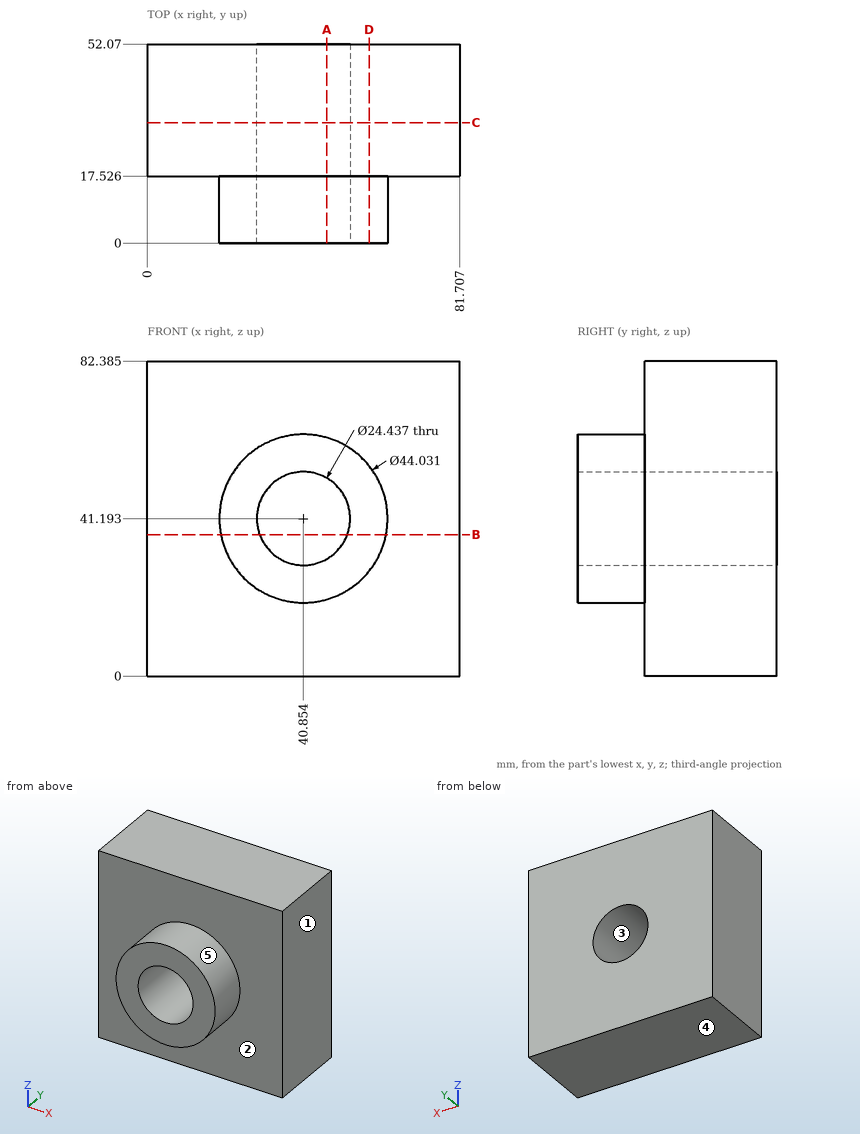
Check sheet for the drawn part. Datum: minimum x, y, z corner. Units: mm. A direction names the side the tool comes from. Round coordinates to 2 decimals unless told otherwise and drop trailing zeros. Order: outer loops, then holes, each group sorted by start corner. A loop starts at its lowest first (then second) coordinate and runs counter-clockwise, first axis right, second up. Notation, with made-up numbers: M 50,50.25 L 99,50.25 A33 ccw 99,80.25 Z; hole C -5,-6.75 d4. An arc over 180 degrees is marked long. Write each question's results on one line, items separated by ' | '. Start each with the question number.
1. Cross-section at B-B on z = 37. Record the boundary of the cut face in (x, y).
2. Cross-section at C-C on y = 31.5. Record the boundary of the cut face in (x, z) (1 decimal).
3. Go/stop test with flat-tipped pins: P1, Ø12, axis at x = 29.5, y = 5.5, coming from the +Z side; P2, Ø10, axis at x = 49.5, z = 40, coming from the -Y side; P3, Ø2, axis at x = 32, y = 11, coming from the -Z side (1 decimal); P4, Ø1, axis at x = 50, z = 63.5, coming from the -Y side. Record where each tip stops, or that it passes through.
4. Cross-section at A-A on x = 47. Record the boundary of the cut face in (y, z) (1 decimal).
5. Material ranges on L1, parallel to Y at x = 57, z = 21; L2, parallel to Z at x = 50, y = 13 (1 decimal); L3, parallel to X at y = 13, z = 46.5, recorded low to high. Write a range as from..to.
6. Set-up check for the marked faces 1 and 2: record each of +Z, -Z, +X, -X, +Y, -Y from which the full face is reachable in a straight line by a thin tool's end or side.
7. Draft check along Z on the marked faces 3, 4 and 5. Enter one of: pulls with the +Z half, pulls with the -Z half, needs draft (parallel to the pull), parting line crosses it, or undercut.
8. Cross-section at D-D on x = 58. Record the boundary of the cut face in (y, z) (1 decimal), plus the area to 3 significant figures.
Resolved:
1) outline: M 0,17.53 L 19.24,17.53 L 19.24,0 L 29.38,0 L 29.38,52.07 L 0,52.07 Z; M 52.33,0 L 62.47,0 L 62.47,17.53 L 81.71,17.53 L 81.71,52.07 L 52.33,52.07 Z
2) outline: M 0,0 L 81.7,0 L 81.7,82.4 L 0,82.4 Z; hole C 40.9,41.2 d24.4
3) P1: z = 62.55 | P2: y = 0 | P3: z = 20.6 | P4: y = 17.53
4) outline: M 0,20.1 L 17.5,20.1 L 17.5,0 L 52.1,0 L 52.1,30.6 L 0,30.6 Z; M 0,51.8 L 52.1,51.8 L 52.1,82.4 L 17.5,82.4 L 17.5,62.3 L 0,62.3 Z
5) L1: 17.53..52.07 | L2: 21.2..33.1, 49.3..61.2 | L3: 19.49..29.85, 51.86..62.22
6) face 1: +Z, -Z, +X, +Y, -Y | face 2: -Y
7) face 3: undercut | face 4: pulls with the -Z half | face 5: parting line crosses it
8) outline: M 0,27.4 L 17.5,27.4 L 17.5,0 L 52.1,0 L 52.1,82.4 L 17.5,82.4 L 17.5,55 L 0,55 Z | area: 3,330 mm2
